Here's the drawing with two shaded views (mm, measured from the low corner). I have some questions. A direction names the side the tool comes from. Coordinates: 2 decimals unless noted, no trailing zeros. Write each loop counter-clockwise with the first axis right and the second up, starting at its lowest first coordinate (ties: lowest second). Pieces come first, ordered by that corner, then holes.
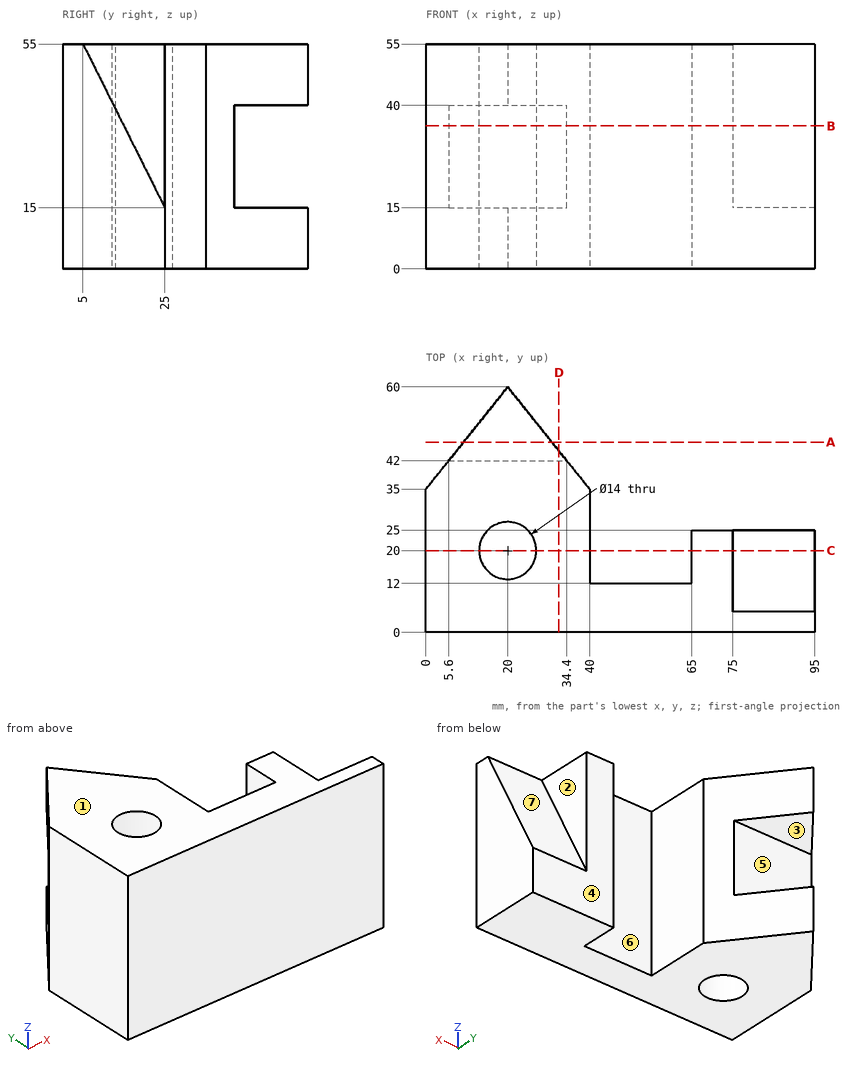
Item 1: If we mould it in two halves opening along Z, with no side actions, what happens to the marked faces 1, 2 and 3? For each: released by +Z, released by -Z, zero draft, split by the parting line, or undercut.
Item 2: I want a section at D-D, the plane x = 32.5. List the corners of the cut face in (y, z) for me (3 decimals), then the cut area to 3 significant figures.
Item 3: I want a section at A-A, the plane y = 46.5. List the corners of the cut face in (x, z) for me.
Item 4: I want a section at C-C, the plane y = 20. List the corners of the cut face in (x, z) for me, then the cut area to 3 significant figures.
Item 5: Which directions (+Z, -Z, +X, -X, +Y, -Y) give clear straight access to the entire face, cutting with the end or side of a thin tool? Please do the marked faces 4, 5, 6 and 7.
Item 6: If I drill on line 1 along Z through (x, y) = (26, 48); line 2 along Y through (x, z) = (20, 14); line 3 along Y through (x, z) = (19.5, 25.5), over which ranges is the centre line in solid material (lowest first)?
Item 7: I want a section at B-B, the plane z = 35. List the corners of the cut face in (x, y) for me, then the cut area to 3 significant figures.
Item 8: Will these pins go through, and if not, where does the flat tip stop? pin 1 Ø2 at (y, z) = (34, 20) entering from +X; pin 2 Ø12.5 at (x, z) = (52, 25.5) entering from +Y; pin 3 Ø11 at (x, y) = (20, 20) entering from -Z; pin 4 Ø1 at (x, z) = (26, 7) entering from +Y (3 decimals).
Taken from the geometry:
1. face 1: released by +Z
1. face 2: zero draft
1. face 3: undercut
2. outline: (0, 0) - (44.375, 0) - (44.375, 15) - (42, 15) - (42, 40) - (44.375, 40) - (44.375, 55) - (0, 55) - close
2. area: 2,380 mm2
3. outline: (9.2, 0) - (30.8, 0) - (30.8, 15) - (9.2, 15) - close; (9.2, 40) - (30.8, 40) - (30.8, 55) - (9.2, 55) - close
4. outline: (0, 0) - (13, 0) - (13, 55) - (0, 55) - close; (27, 0) - (40, 0) - (40, 55) - (27, 55) - close; (65, 0) - (95, 0) - (95, 25) - (75, 25) - (75, 55) - (65, 55) - close
4. area: 2,480 mm2
5. face 4: +Z, -Z, +X, +Y
5. face 5: +X, -X, +Y
5. face 6: +Z, -Z, +Y
5. face 7: +Z, +X, +Y
6. line 1: z = 0 to 15, 40 to 55
6. line 2: y = 0 to 13, 27 to 60
6. line 3: y = 0 to 13.02, 26.98 to 42
7. outline: (0, 0) - (95, 0) - (95, 15) - (75, 15) - (75, 25) - (65, 25) - (65, 12) - (40, 12) - (40, 35) - (34.4, 42) - (5.6, 42) - (0, 35) - close; hole circle Ø14 at (20, 20)
7. area: 2,340 mm2
8. pin 1: stops at x = 40
8. pin 2: stops at y = 12
8. pin 3: passes through
8. pin 4: stops at y = 53.125
